The listing builds one solid part. Answer for the finished solid, in the listing's coordinates (mm). Face numbers are marked on the shaded views. A direction names the side the tool comes from. Round coordinates to 2 decimals unless told otherwise and drop trailing zeros. Write each loop counter-clockwise with the first axis right and the second up, starting at its lowest first coordinate (ties: lowest second). Pieces come first, ordered by that corner, then holes. Notation, with made-up numbers: M 4.5,5.5 L 20.5,5.5 A22 cw 20.5,12.5 Z; hole C -32.5,-19 d7. An arc over 180 degrees is marked long. Put each result on its own line as item: value. Start each with the question number.
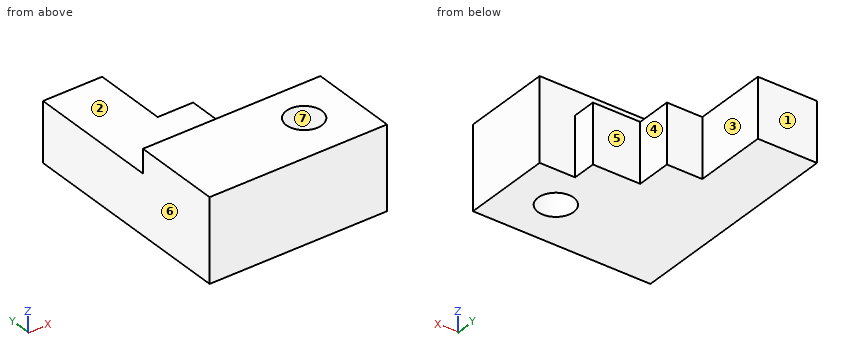
```python
from build123d import *

# Parameters (mm, degrees)
CROQUIS2_W              = 60
CROQUIS2_H              = 30
SALIENTE_EXTRUIR1_DEPTH = 28
SALIENTE_EXTRUIR2_DEPTH = 20
CROQUIS5_R              = 6
CORTAR_EXTRUIR1_DEPTH   = 29


with BuildPart() as part:
    # Croquis2 → Saliente-Extruir1 (new body)
    with BuildSketch(Plane.XY):
        with Locations((-30, 15)):
            Rectangle(CROQUIS2_W, CROQUIS2_H)
    extrude(amount=SALIENTE_EXTRUIR1_DEPTH)

    # Croquis2_4 → Saliente-Extruir2 (add)
    with BuildSketch(Plane.XY):
        Polygon((-60, 75), (-60, 30), (-12, 30), (-12, 38), (-28, 38), (-28, 50), (-40, 50), (-40, 75), align=None)
    extrude(amount=SALIENTE_EXTRUIR2_DEPTH)

    # Croquis5 → Cortar-Extruir1 (cut, through all)
    with BuildSketch(Plane.XY.offset(28)):
        with Locations((-16, 16)):
            Circle(CROQUIS5_R)
    extrude(amount=-CORTAR_EXTRUIR1_DEPTH, mode=Mode.SUBTRACT)


solid = part.part
```
Item 1: Which of the six approach directions +Z, -Z, +X, -X, +Y, -Y give full straight-line access (tool end or side, diameter ignored) to the marked faces 1, 2 and 3?
Item 2: Flat-ended cylindrical pins translate along their axes: pin 1 (10 mm diameter, centred on x = -26, z = 22, fed in from -Y); pin 2 (9.5 mm diameter, centred on x = -33, z = 13, fed in from +Y); pin 3 (10 mm diameter, centred on y = 63, z = 9, fed in from +X); pin 4 (13 mm diameter, centred on x = -17.5, z = 7.5, fed in from +Y). Find the tip coordinate at first contact, or state that the pin passes through.
Item 3: Section C-C (z = 22.25) is taken. Give the vertices of the cut face in (x, y), and give its area (3 significant figures).
Item 4: Consider line 1 along Y through (x, z) = (-16, 21); line 2 along Y through (x, z) = (-40, 23); line 3 along Y through (x, z) = (-39.5, 3.5). Determine where each line is inside the solid, lowest interval first. Write a range as [from, to].
Item 5: Section D-D (x = -53) is taken. Give the vertices of the cut face in (y, z).
Item 6: Section B-B (x = -16) is taken. Give the vertices of the cut face in (y, z).
Item 7: Section A-A (y = 16) is taken. Give the vertices of the cut face in (x, z), and give its area (3 significant figures).
Item 8: Determine the mould class of the marked faces 4, 5, 6 and 7 for opening direction X: released by +X, released by -X, zero draft, split by the parting line, or undercut.
Output values:
1. face 1: +Z, -Z, +X, -X, +Y
1. face 2: +Z, +X, -X, +Y
1. face 3: +Z, -Z, +X, +Y
2. pin 1: stops at y = 0
2. pin 2: stops at y = 50
2. pin 3: stops at x = -40
2. pin 4: stops at y = 38
3. outline: M -60,0 L 0,0 L 0,30 L -60,30 Z; hole C -16,16 d12
3. area: 1,690 mm^2
4. line 1: y = [0, 10], [22, 30]
4. line 2: y = [0, 30]
4. line 3: y = [0, 50]
5. outline: M 0,0 L 75,0 L 75,20 L 30,20 L 30,28 L 0,28 Z
6. outline: M 0,0 L 10,0 L 10,28 L 0,28 Z; M 22,0 L 38,0 L 38,20 L 30,20 L 30,28 L 22,28 Z
7. outline: M -60,0 L -22,0 L -22,28 L -60,28 Z; M -10,0 L 0,0 L 0,28 L -10,28 Z
7. area: 1,340 mm^2
8. face 4: released by +X
8. face 5: zero draft
8. face 6: released by -X
8. face 7: undercut
